from build123d import *

# Parameters (mm, degrees)
CROQUIS1_W                 = 22
CROQUIS1_H                 = 100.5
CROQUIS1_R                 = 1.75
CROQUIS1_R_2               = 1
CROQUIS1_W_2               = 13
CROQUIS1_H_2               = 23
CROQUIS1_W_3               = 5.5
CROQUIS1_H_3               = 5
SALIENTE_EXTRUIR1_DEPTH    = 35
CORTAR_EXTRUIR2_DEPTH      = 100.494974747
CORTAR_EXTRUIR2_DEPTH_BACK = 100.494974747


with BuildPart() as part:
    # Croquis1 → Saliente-Extruir1 (new, symmetric)
    with BuildSketch(Plane(origin=(0, 0, 0), x_dir=(0, 0, -1), z_dir=(1, 0, 0))):
        with Locations((0, 40.25)):
            Rectangle(CROQUIS1_W, CROQUIS1_H)
        with Locations((-8.75, 20.5)):
            Circle(CROQUIS1_R, mode=Mode.SUBTRACT)
        with Locations((8.75, 20.5)):
            Circle(CROQUIS1_R, mode=Mode.SUBTRACT)
        with Locations((0, 85.25)):
            Circle(CROQUIS1_R_2, mode=Mode.SUBTRACT)
        with Locations((0, 57.75)):
            Circle(CROQUIS1_R_2, mode=Mode.SUBTRACT)
        with BuildLine():
            Line((-6.565214453, 4.571428571), (-1.641303613, 11.642857143))
            ThreePointArc((-1.641303613, 11.642857143), (0, 12.5), (1.641303613, 11.642857143))
            Line((1.641303613, 11.642857143), (6.565214453, 4.571428571))
            ThreePointArc((6.565214453, 4.571428571), (0, -8), (-6.565214453, 4.571428571))
        make_face(mode=Mode.SUBTRACT)
        with Locations((0, 71.5)):
            Rectangle(CROQUIS1_W_2, CROQUIS1_H_2, mode=Mode.SUBTRACT)
        with Locations((0, 29)):
            Rectangle(CROQUIS1_W_3, CROQUIS1_H_3, mode=Mode.SUBTRACT)
    extrude(amount=SALIENTE_EXTRUIR1_DEPTH, both=True)

    # Croquis2 → Cortar-Extruir2 (cut, two sides: drawn at the far end of the back side and taken through both)
    with BuildSketch(Plane.XY.offset(11).offset(-CORTAR_EXTRUIR2_DEPTH_BACK)):
        Polygon((32.5, -262.128065288), (32.5, -10), (32.5, 88), (-32.5, 88), (-32.5, -10), (-32.5, -262.128065288), (-32.5, -766.384195863), (32.5, -766.384195863), align=None)
    extrude(amount=CORTAR_EXTRUIR2_DEPTH + CORTAR_EXTRUIR2_DEPTH_BACK, mode=Mode.SUBTRACT)


solid = part.part
Source: CAD feature listing. Evaluate the final solid. Frame: model axes, mm. A direction names the side the tool comes from. Coordinates: 2 decimals unless noted, no trailing zeros. Order: outer loops, then holes, each group sorted by start corner. A loop starts at its lowest first (then second) coordinate and runs counter-clockwise, first axis right, second up. Notation, with made-up numbers: M 51,77 L 68,77 A13 cw 68,83 Z; hole C 64,56.25 d10. An arc over 180 degrees is marked long. Write each question's results on one line, items separated by ' | '. Start each with the question number.
Item 1: Cut plane B-B (z = -9.25). Return loops of the section in (x, y), and give its area (3 significant figures).
Item 2: Set-up query: faces 1 (the face through (0, 90.5, 0)), 2 (the face through (0, 88, 0)), 3 (the face through (33.768, 8.058, 4.138)). Return all of +Z, -Z, +X, -X, +Y, -Y with unobstructed straight access to the full face (end or side cutting, diameter ignored); none if empty.
Item 3: Cut plane C-C (y = 25.5). Return loops of the section in (x, z).
Item 4: Cut plane D-D (y = 0). Return loops of the section in (x, z).
Item 5: Cut plane A-A (y = 78). Return loops of the section in (x, z).
Item 6: First-contact query: pin 1 Ø4.5 at (y, z) = (20.5, 8.75) entering from -X; pin 2 Ø6 at (x, z) = (21, 6.5) entering from -Y. Flat tips, straight axial feed; report the tip coordinate or a pass-through.
Item 7: Draft query along Z for faces 4 (the face through (-34, 71, 6.5)), 5 (the face through (-32.5, 40, 0)). Return one class per face: pulls with the +Z half, pulls with the -Z half, needs draft (parallel to the pull), parting line crosses it, or undercut.
Item 8: Line query: probe 1 along Z at (x, y) = (33.15, 20.5); probe 2 along Z at (x, y) = (33.9, 85.25); probe 3 along X at (y, z) = (86, -6.25). Output: solid intervals per line, ascending.
Checked values:
1) outline: M -35,-10 L -32.5,-10 L -32.5,18.82 L -35,18.82 Z; M -35,22.18 L -32.5,22.18 L -32.5,88 L 32.5,88 L 32.5,22.18 L 35,22.18 L 35,90.5 L -35,90.5 Z; M 32.5,-10 L 35,-10 L 35,18.82 L 32.5,18.82 Z | area: 648 mm2
2) face 1: +Z, -Z, +X, -X, +Y | face 2: +Z, -Z, -Y | face 3: +X, -X
3) outline: M -35,-11 L -32.5,-11 L -32.5,11 L -35,11 Z; M 32.5,-11 L 35,-11 L 35,11 L 32.5,11 Z
4) outline: M -35,-11 L -32.5,-11 L -32.5,-8 L -35,-8 Z; M -35,8 L -32.5,8 L -32.5,11 L -35,11 Z; M 32.5,-11 L 35,-11 L 35,-8 L 32.5,-8 Z; M 32.5,8 L 35,8 L 35,11 L 32.5,11 Z
5) outline: M -35,-11 L -32.5,-11 L -32.5,-6.5 L -35,-6.5 Z; M -35,6.5 L -32.5,6.5 L -32.5,11 L -35,11 Z; M 32.5,-11 L 35,-11 L 35,-6.5 L 32.5,-6.5 Z; M 32.5,6.5 L 35,6.5 L 35,11 L 32.5,11 Z
6) pin 1: stops at x = -35 | pin 2: stops at y = 88
7) face 4: undercut | face 5: needs draft
8) probe 1: z = -11 to -10.5, -7 to 7, 10.5 to 11 | probe 2: z = -11 to -1, 1 to 11 | probe 3: x = -35 to -32.5, 32.5 to 35
